Input: part model. Units: mm. Frame: model coordinates. A direction names the side the tool comes from. Round coordinates to 2 decimals unless told otherwise and drop trailing zeros. Order: outer loops, then holes, each group sorted by start corner. A loop starts at its lowest first (then second) coordinate and runs counter-clockwise, first axis right, second up. Notation, with made-up numbers: (72, 60) -> (90, 60) arc R17 ccw to (90, 74) -> close; hole circle Ø1 at (30.25, -1). An arc over 180 degrees is marked (long way). Use a Markdown table: item, result.
from build123d import *

# Parameters (mm, degrees)
ESTRUSIONE_ESTRUSIONE1_DEPTH  = 7
TAGLIO_ESTRUSIONE1_DEPTH      = 6
SCHIZZO3_W                    = 16
SCHIZZO3_H                    = 7
ESTRUSIONE_ESTRUSIONE2_DEPTH  = 49.55
SCHIZZO6_W                    = 28.452677992
SCHIZZO6_H                    = 5
ESTRUSIONE_ESTRUSIONE5_DEPTH  = 5
SCHIZZO7_W                    = 28.5
SCHIZZO7_H                    = 5
ESTRUSIONE_ESTRUSIONE6_DEPTH  = 5
TAGLIO_ESTRUSIONE8_DEPTH      = 52.802078251
TAGLIO_ESTRUSIONE8_DEPTH_BACK = 52.802078251
RACCORDO1_R                   = 2


with BuildPart() as part:
    # Schizzo1 → Estrusione-Estrusione1 (new body)
    with BuildSketch(Plane.XY):
        Polygon((-15.909106105, 13.642580206), (-5.669705551, 20.812285661), (22.75100687, -19.776698134), (12.511606316, -26.946403588), align=None)
    extrude(amount=ESTRUSIONE_ESTRUSIONE1_DEPTH)

    # Schizzo1<3> → Taglio-Estrusione1 (cut)
    with BuildSketch(Plane.XY):
        Polygon((-14.500401843, 14.443682773), (13.695602758, -25.824384995), (13.204111531, -26.168530857), (-14.991893069, 14.099536911), align=None)
        Polygon((-6.36666227, 20.087622092), (-6.858153497, 19.74347623), (21.304903969, -20.477538154), (21.796395196, -20.133392292), align=None)
    extrude(amount=TAGLIO_ESTRUSIONE1_DEPTH, mode=Mode.SUBTRACT)

    # Schizzo3 → Estrusione-Estrusione2 (add)
    with BuildSketch(Plane(origin=(16.77686077, -23.959840268, 0), x_dir=(-0.8191520442889922, -0.5735764363510456, 0), z_dir=(0.5735764363510455, -0.8191520442889921, 0))):
        with Locations((-15.293085749, -3.5)):
            Rectangle(SCHIZZO3_W, SCHIZZO3_H)
    extrude(amount=-ESTRUSIONE_ESTRUSIONE2_DEPTH)

    # Schizzo6 → Estrusione-Estrusione5 (add)
    with BuildSketch(Plane(origin=(16.77686077, -23.959840268, 0), x_dir=(-0.8191520442889922, -0.5735764363510456, 0), z_dir=(0.5735764363510455, -0.8191520442889921, 0))):
        with Locations((-9.019424745, -4.5)):
            Rectangle(SCHIZZO6_W, SCHIZZO6_H)
    extrude(amount=ESTRUSIONE_ESTRUSIONE5_DEPTH)

    # Schizzo7 → Estrusione-Estrusione6 (add)
    with BuildSketch(Plane(origin=(-11.643851652, 16.629143527, 0), x_dir=(0.8191520442889902, 0.5735764363510484, 0), z_dir=(-0.5735764363510484, 0.8191520442889902, 0))):
        with Locations((9.043085749, -4.5)):
            Rectangle(SCHIZZO7_W, SCHIZZO7_H)
    extrude(amount=ESTRUSIONE_ESTRUSIONE6_DEPTH)

    # Schizzo8 → Taglio-Estrusione8 (cut, two sides: drawn at the far end of the back side and taken through both)
    with BuildSketch(Plane(origin=(0, 0, 2), x_dir=(-1, 0, 0), z_dir=(0, 0, -1)).offset(-TAGLIO_ESTRUSIONE8_DEPTH_BACK)):
        with BuildLine():
            Line((-33.988775508, -12.923786256), (-15.062626046, -26.452245662))
            ThreePointArc((-15.062626046, -26.452245662), (-14.714599039, -28.544822352), (-16.807175729, -28.892849359))
            Line((-16.807175729, -28.892849359), (-35.733325191, -15.364389953))
            ThreePointArc((-35.733325191, -15.364389953), (-36.081352198, -13.271813263), (-33.988775508, -12.923786256))
        make_face()
        with BuildLine():
            Line((-2.62416195, 31.45957899), (16.301987512, 17.931119584))
            ThreePointArc((16.301987512, 17.931119584), (16.650014519, 15.838542895), (14.55743783, 15.490515888))
            Line((14.55743783, 15.490515888), (-4.368711632, 29.018975294))
            ThreePointArc((-4.368711632, 29.018975294), (-4.71673864, 31.111551983), (-2.62416195, 31.45957899))
        make_face()
    extrude(amount=TAGLIO_ESTRUSIONE8_DEPTH + TAGLIO_ESTRUSIONE8_DEPTH_BACK, mode=Mode.SUBTRACT)

    # Raccordo1
    raccordo1_edges = [part.edges().sort_by_distance(p)[0] for p in [
        (15.379488498, -31.04216381, 4.5),
        (38.686557841, -14.722378162, 4.5),
        (-18.776988287, 17.738340428, 4.5),
        (4.568844976, 34.085268864, 4.5),
    ]]
    fillet(raccordo1_edges, radius=RACCORDO1_R)


solid = part.part
1) Cut plane C-C on y = -19. Return loops of the section in (x, z).
Results found:
| item | result |
|---|---|
| outline | (6.95, 0) -> (8.18, 0) -> (8.18, 6) -> (8.92, 6) -> (8.92, 0) -> (20.27, 0) -> (20.27, 6) -> (21, 6) -> (21, 0) -> (23.86, 0) -> (23.86, 2) -> (25.49, 2) -> (25.49, 7) -> (6.95, 7) -> close; (30.65, 2) -> (32.58, 2) -> (32.58, 7) -> (30.65, 7) -> close |
2) Pin query (flat end, axial travel): pin 1 Ø1 at (x, z) = (-1.5, 4.5) entering from +Y; pin 2 Ø1 at (x, z) = (24.5, 3) entering from -Y; pin 3 Ø4 at (y, z) = (-22.5, 5) entering from -X. Return the tip coordinate at first contact, or that it passes through.
Results found:
| item | result |
|---|---|
| pin 1 | stops at y = 30.19 |
| pin 2 | stops at y = -25.01 |
| pin 3 | stops at x = 8 |
3) Cut plane A-A on z = 4. Return loops of the section in (x, y), and give its area (3 significant figures).
Results found:
| item | result |
|---|---|
| outline | (-17.63, 16.1) -> (14.23, -29.4) arc R2 ccw to (17.02, -29.9) -> (37.05, -15.87) arc R2 ccw to (37.54, -13.08) -> (35.82, -10.63) -> (35.86, -10.6) -> (5.72, 32.45) arc R2 ccw to (2.93, 32.94) -> (-17.14, 18.89) arc R2 ccw to start; hole (-16.3, 17.93) arc R1.5 ccw to (-14.56, 15.49) -> (4.37, 29.02) arc R1.5 ccw to (2.62, 31.46) -> close; hole (-14.99, 14.1) -> (13.2, -26.17) -> (13.7, -25.82) -> (-14.5, 14.44) -> close; hole (-6.86, 19.74) -> (21.3, -20.48) -> (21.8, -20.13) -> (-6.37, 20.09) -> close; hole (15.06, -26.45) arc R1.5 ccw to (16.81, -28.89) -> (35.73, -15.36) arc R1.5 ccw to (33.99, -12.92) -> close |
| area | 1,480 mm² |
4) Cut plane D-D on y = 7. Return loops of the section in (x, z).
Results found:
| item | result |
|---|---|
| outline | (-11.26, 0) -> (-10.02, 0) -> (-10.02, 6) -> (-9.29, 6) -> (-9.29, 0) -> (2.06, 0) -> (2.06, 6) -> (2.8, 6) -> (2.8, 0) -> (23.53, 0) -> (23.53, 7) -> (-11.26, 7) -> close |
5) Cut plane B-B on x = 32.5. Return loops of the section in (y, z).
Results found:
| item | result |
|---|---|
| outline | (-19.05, 2) -> (-17.68, 2) -> (-17.68, 7) -> (-19.05, 7) -> close; (-13.99, 2) -> (-12.95, 2) -> (-12.95, 0) -> (-5.8, 0) -> (-5.8, 7) -> (-13.99, 7) -> close |
6) Set-up query: faces 4 (the flat face through (-7, 25, 2)), 5 (the flat face through (-6.706, 24.79, 4.535)), 6 (the flat face through (36.67, -11.84, 4.54)), 7 (the flat face through (-0.6, -5.41, 2.96)), 8 (the flat face through (10, 1, 0)). Return all of +Z, -Z, +X, -X, +Y, -Y with unobstructed straight access to the full face (end or side cutting, diameter ignored); none if empty.
Results found:
| item | result |
|---|---|
| face 4 | -Z, -X, +Y |
| face 5 | +Z, -Z |
| face 6 | +Z, -Z, +X, +Y |
| face 7 | -Z |
| face 8 | -Z, +X, -X, +Y, -Y |
7) Line query: L1, parallel to X at y = -23.5, z = 5.5; L2, parallel to X at y = -9, z = 4.25; L3, parallel to Y at x = 20.5, z = 2.5. Output: solid intervals per line, ascending. Write a range as [from, to].
Results found:
| item | result |
|---|---|
| L1 | x = [10.1, 11.34], [12.07, 19.19], [24.35, 26.15] |
| L2 | x = [-0.05, 1.18], [1.92, 13.27], [14, 34.74] |
| L3 | y = [-27.46, -26.25], [-22.57, -19.33], [-18.28, 11.33] |
8) Pull-direction query (X, two-part tool) for faces 1 (the flat face through (7.91, -0.3, 2.96)), 2 (the flat face through (10, 1, 7)), 3 (the flat face through (-7.245, 25.813, 4.465)); classes: +X half, -X half, draft (parallel to the pull), parting line (faces both ways), or undercut.
Results found:
| item | result |
|---|---|
| face 1 | undercut |
| face 2 | draft |
| face 3 | -X half |
